Check sheet for the modelled part. Datum: model origin and axes. Units: mm. A direction names the side the tool comes from. Give positions to 0.01 mm unless a question says otherwise; leave off trailing zeros. Write each loop counter-clockwise with the first axis right and the second up, starting at its lowest first coordinate (ties: lowest second). Pieces come first, ordered by that corner, then holes. Notation, with made-up numbers: M 63.5,43 L 92.5,43 A27 ccw 92.5,63 Z; hole C 53.25,-39.5 d5. An arc over 180 degrees is marked long. Write item = value, one per line. Start each with the question number.
1) Draft check along Y on faces 1 (the face through (-20.674, -0.897, -1.471)), 2 (the face through (-21, -7, 0)), 3 (the face through (-6.431, -6.083, 6.633)), 4 (the face through (-19.851, 2.613, 10.068)). Enter one of: pulls with the +Y half, pulls with the -Y half, needs draft (parallel to the pull), parting line crosses it, or undercut.
2) Set-up check for faces 5 (the face through (-67, 0, -8)), 6 (the face through (-62, -8, 0)), 7 (the face through (-59, 5, -5.2)), 8 (the face through (-11, 7, 7)), 9 (the face through (-67.6, -4.9, 5)): record each of +Z, -Z, +X, -X, +Y, -Y from which the full face is reachable in a straight line by a thin tool's end or side.
3) Sectioned sample at D-D, the plane y = 3.5. Count the separate pieces of the cut face and the enclosed holes in it, then the cut area to 3 significant figures.
4) Sectioned sample at B-B, the plane y = -10. Record the cut outline in (x, z), then the cut area to 3 significant figures.
5) Sectioned sample at A-A, the plane x = -63. Record the cut outline in (y, z).
6) Gauge pin test, flat ends, axial feed: pin 1 (5 mm diameter, centred on x = -47.5, z = -8, fed in from +Y); pin 2 (8 mm diameter, centred on x = -30.5, y = 4, fed in from -Z); pin 3 (8 mm diameter, centred on x = -12.5, z = 3, fed in from +Y); pin 4 (10 mm diameter, centred on x = -55.5, z = -14.5, fed in from +Y). Record the tip position at first contact, or that the pin passes through.
7) Scan lines: L1, parallel to X at y = -10, z = 10; L2, parallel to X at y = 7, z = 1.5; L3, parallel to Y at x = -21, z = -10. Record each from-to range of solid material in increasing order.
8) Sectioned sample at C-C, the plane z = -14. Record the cut outline in (x, y), then the cut area to 3 significant figures.
from build123d import *

# Parameters (mm, degrees)
CUT_EXTRUDE_1_DEPTH      = 82.092539731
CUT_EXTRUDE_1_DEPTH_BACK = 82.092539731
SKETCH_2_R               = 3
PATTERN_CIRCULAR_1_COUNT = 2
PATTERN_CIRCULAR_1_ANGLE = 60
SKETCH_6_OUTSIDE_W       = 60.93
SKETCH_6_OUTSIDE_H       = 60.704
CUT_EXTRUDE_2_DEPTH      = 17
HOLE_WIZARD_M61_D        = 5
CUT_EXTRUDE_3_DEPTH      = 10


with BuildPart() as part:
    # Эскиз1 → Повернуть1 (revolve)
    with BuildSketch(Plane.XY, mode=Mode.PRIVATE) as revolve_1_sk:
        with BuildLine():
            Line((0, 0), (0, 8))
            Line((0, 8), (-1.732050808, 9))
            Line((-1.732050808, 9), (-11, 9))
            Line((-11, 9), (-11, 17.320508076))
            ThreePointArc((-11, 17.320508076), (-21, 20), (-31, 17.320508076))
            Line((-31, 17.320508076), (-31, 9))
            Line((-31, 9), (-57.267949192, 9))
            Line((-57.267949192, 9), (-59, 8))
            Line((-59, 8), (-75, 8))
            Line((-75, 8), (-76, 7))
            Line((-76, 7), (-76, 0))
            Line((-76, 0), (0, 0))
        make_face()
    revolve(revolve_1_sk.sketch.rotate(Axis((0, 0, 0), (-1, 0, 0)), 90), axis=Axis((0, 0, 0), (-1, 0, 0)))

    # Эскиз2 → Вырез-Вытянуть1 (cut, two sides: drawn at the far end of the back side and taken through both)
    with BuildSketch(Plane.XY.offset(-CUT_EXTRUDE_1_DEPTH_BACK)):
        with Locations(Location((-21, -10, 0), (0, 0, 235.677064265))):
            Circle(SKETCH_2_R)
    extrude(amount=CUT_EXTRUDE_1_DEPTH + CUT_EXTRUDE_1_DEPTH_BACK, mode=Mode.SUBTRACT)

    # Эскиз4 → Диаметр отверстия Ø6.0 (6)1 (revolve, cut)
    with BuildSketch(Plane(origin=(-21, 20, 0), x_dir=(0, 0, 1), z_dir=(1, 0, 0))):
        Polygon((0, 0), (0, 21.802581857), (3, 20), (3, 0), align=None)
    hole_wizard_6_0_6_1 = revolve(axis=Axis((-21, 20, 0), (0, -1, 0)), mode=Mode.SUBTRACT)

    # Круговой массив1: Диаметр отверстия Ø6.0 (6)1 ×2 about axis
    pattern_circular_1_axis = Axis((0, 0, 0), (1, 0, 0))
    for i in range(1, PATTERN_CIRCULAR_1_COUNT):
        add(hole_wizard_6_0_6_1.rotate(pattern_circular_1_axis, i * PATTERN_CIRCULAR_1_ANGLE / (PATTERN_CIRCULAR_1_COUNT - 1)), mode=Mode.SUBTRACT)

    # Эскиз6 outside → Вырез-Вытянуть2 (cut)
    with BuildSketch(Plane.ZY.offset(76)):
        with Locations((0, -0.113)):
            Rectangle(SKETCH_6_OUTSIDE_W, SKETCH_6_OUTSIDE_H)
        Polygon((-9.899494937, 0), (0, 9.899494937), (9.899494937, 0), (0, -9.899494937), align=None, mode=Mode.SUBTRACT)
    extrude(amount=-CUT_EXTRUDE_2_DEPTH, mode=Mode.SUBTRACT)

    # Отверстие обработанное метчиком M61 (through all)
    with Locations(Plane(origin=(0, 10, 0), x_dir=(1, 0, 0), z_dir=(0, 1, 0))):
        with Locations((-68, 0)):
            Hole(HOLE_WIZARD_M61_D / 2)

    # Эскиз11 → Вырез-Вытянуть3 (cut)
    with BuildSketch(Plane(origin=(0, 10, 0), x_dir=(1, 0, 0), z_dir=(0, 1, 0))):
        Polygon((-76, 0.5), (-75.5, 0), (-76, -0.5), align=None)
    extrude(amount=-CUT_EXTRUDE_3_DEPTH, mode=Mode.SUBTRACT)


solid = part.part
Data:
q1.face_1 = pulls with the +Y half
q1.face_2 = undercut
q1.face_3 = parting line crosses it
q1.face_4 = undercut
q2.face_5 = -Z, -X
q2.face_6 = -X, -Y
q2.face_7 = -Z, -X, +Y
q2.face_8 = +X
q2.face_9 = +Z, -X, -Y
q3.separate_pieces = 1
q3.enclosed_holes = 2
q3.area = 1,520 mm2
q4.outline = M -31,-14.14 A17.32 ccw -24,-17.06 L -24,17.06 A17.32 ccw -31,14.14 Z; M -18,-17.06 A17.32 ccw -11,-14.14 L -11,14.14 A17.32 ccw -18,17.06 Z
q4.area = 445 mm2
q5.outline = M -7.69,-2.21 L -2.21,-7.69 A8 ccw 2.21,-7.69 L 7.69,-2.21 A8 ccw 7.69,2.21 L 2.21,7.69 A8 ccw -2.21,7.69 L -7.69,2.21 A8 ccw Z
q6.pin_1 = 7.12
q6.pin_2 = -18.98
q6.pin_3 = 19.36
q6.pin_4 = through
q7.L1 = -31 to -24, -18 to -11
q7.L2 = -75.84 to -70, -66 to -23.6, -18.4 to 0
q7.L3 = -17.32 to -13, -7 to 17.32
q8.outline = M -31,-10.2 A14.28 ccw -11,-10.2 L -11,10.2 A14.28 ccw -31,10.2 Z; hole C -21,-10 d6
q8.area = 492 mm2
